from build123d import *

# Parameters (mm, degrees)
SKETCH1_R           = 3.0861
SKETCH1_R_2         = 2.29235
BOSS_EXTRUDE1_DEPTH = 6.35


with BuildPart() as part:
    # Sketch1 → Boss-Extrude1 (new body)
    with BuildSketch(Plane.XY):
        with BuildLine():
            Line((9.317684399, -23.927461165), (15.621766017, -30.474222957))
            add(Edge.make_bspline(
                [(15.621766017, -30.474222957), (29.448816856, -35.495722543), (24.952941844, -21.488942011)],
                knots=[0, 0, 0, 1, 1, 1], degree=2))
            Line((24.952941844, -21.488942011), (17.141687262, -13.376987542))
            ThreePointArc((17.141687262, -13.376987542), (42.59986543, 14.894415901), (71.784823307, 39.299934171))
            Line((71.784823307, 39.299934171), (79.625725522, 31.157190761))
            add(Edge.make_bspline(
                [(79.625725522, 31.157190761), (93.452776362, 26.135691176), (88.956901349, 40.142471708)],
                knots=[0, 0, 0, 1, 1, 1], degree=2))
            Line((88.956901349, 40.142471708), (82.612726668, 46.730869976))
            ThreePointArc((82.612726668, 46.730869976), (89.632476194, 51.148612181), (96.784823972, 55.348284892))
            ThreePointArc((96.784823972, 55.348284892), (101.62072272, 72.831932717), (84.137074895, 77.667831466))
            ThreePointArc((84.137074895, 77.667831466), (24.914787096, 33.479112567), (-21.478374368, -24.032597715))
            ThreePointArc((-21.478374368, -24.032597715), (-17.306021838, -41.68636027), (0.347740718, -37.51400774))
            ThreePointArc((0.347740718, -37.51400774), (4.730111543, -30.652996464), (9.317684399, -23.927461165))
        make_face()
        with Locations((18.173165644, -23.786006993)):
            Circle(SKETCH1_R, mode=Mode.SUBTRACT)
        with Locations((95.832484441, 70.337620248)):
            Circle(SKETCH1_R_2, mode=Mode.SUBTRACT)
        with Locations((-13.699424668, -35.344042378)):
            Circle(SKETCH1_R_2, mode=Mode.SUBTRACT)
        Polygon((-8.010879952, -15.218201264), (-2.100930482, -11.788684368), (7.060562914, -20.950177765), (1.150613445, -24.379694661), align=None, mode=Mode.SUBTRACT)
        Polygon((70.118447134, 60.342279832), (75.060785804, 64.722474401), (83.652705921, 55.027887008), (78.71036725, 50.647692439), align=None, mode=Mode.SUBTRACT)
        with Locations((82.177125837, 37.84540285)):
            Circle(SKETCH1_R, mode=Mode.SUBTRACT)
    extrude(amount=BOSS_EXTRUDE1_DEPTH)


solid = part.part
The listing builds one solid part. Answer for the finished solid, in the listing's coordinates (mm). A direction names the side the tool comes from. Give positions to 0.01 mm unless a question says otherwise; leave off trailing zeros. Loops run counter-clockwise (first coordinate to the right, second up) from the corner with the lowest first, then second, coordinate; pieces in that order, holes last. Notation, with made-up numbers: (-26.5, 53) - (17.5, 53) arc R32 ccw to (17.5, 82) - close; hole circle Ø8 at (75.25, 23). An arc over 180 degrees is marked (long way). Answer as a JSON object with one key per item and string values.
1. A cutting plane is placed at B-B (y = -18.5). Write down the section's boundary in (x, z), then the cut area to 3 significant figures.
Determined:
{"outline": "(-17.98, 0) - (-4.73, 0) - (-4.73, 6.35) - (-17.98, 6.35) - close; (4.61, 0) - (22.07, 0) - (22.07, 6.35) - (4.61, 6.35) - close", "area": "195 mm²"}
2. Flat-ended cylindrical pins translate along their axes: pin 1 Ø1.5 at (x, z) = (64, 3.5) entering from +Y; pin 2 Ø4 at (x, y) = (95.83, 70.34) entering from +Z. Find the tip coordinate at first contact, or state that the pin passes through.
Determined:
{"pin 1": "y = 65.67", "pin 2": "through"}
3. For faces 1 (the flat face through (75.65, 35.286, 3.131)), 2 (the cylindrical face through (25.663, 34.197, 3.131)), 3 (the flat face through (79.3, 59.94, 3.13)), 4 (the cylindrical face through (89.533, 51.088, 3.131)), determine the directions among +Z, -Z, +X, -X, +Y, -Y from which every point of the face is accessible in a straight line to the end or side of a thin tool.
Determined:
{"face 1": "+Z, -Z, -Y", "face 2": "+Z, -Z, -X, +Y", "face 3": "+Z, -Z", "face 4": "+Z, -Z, +X"}
4. A cutting plane is placed at C-C (z = 1). Give the number of separate pieces and of enclosed holes in the cut face, then the cut area to 3 significant figures.
Determined:
{"separate pieces": "1", "enclosed holes": "6", "area": "4,270 mm²"}
5. Find the intervals of material crossed by L1, parallel to X at y = -25.5, z = 0.5; L2, parallel to Y at x = 80, z = 2.5; L3, parallel to Y at x = 81, z = 1, in increasing order. Write a range as [from, to].
Determined:
{"L1": "[-22.26, 8.22], [10.83, 15.61], [20.74, 25.92]", "L2": "[31.02, 35.66], [40.03, 51.79], [59.15, 75.28]", "L3": "[30.69, 34.99], [40.7, 52.68], [58.02, 75.86]"}
6. A cutting plane is placed at D-D (x = 35). Write down the section's boundary in (y, z).
Determined:
{"outline": "(7.27, 0) - (42.75, 0) - (42.75, 6.35) - (7.27, 6.35) - close"}
7. A cutting plane is placed at A-A (x = -13.5). Write down the section's boundary in (y, z), then the cut area to 3 significant figures.
Determined:
{"outline": "(-43.26, 0) - (-37.63, 0) - (-37.63, 6.35) - (-43.26, 6.35) - close; (-33.06, 0) - (-11.8, 0) - (-11.8, 6.35) - (-33.06, 6.35) - close", "area": "171 mm²"}
8. For a pull along X with two mould halves and no side action, classify faces 5 (the cylindrical face through (-12.47, -33.41, 3.13)), 6 (the flat face through (4.15, -22.64, 3.13)), 7 (the cylindrical face through (101.757, 72.585, 3.131)), 8 (the flat face through (40, 18, 0)) as pulls with the +X half, pulls with the -X half, needs draft (parallel to the pull), parting line crosses it, or undercut.
Determined:
{"face 5": "undercut", "face 6": "undercut", "face 7": "parting line crosses it", "face 8": "needs draft"}
